The model under review builds one solid part; all positions refer to its coordinate system, in mm. A direction names the side the tool comes from. Coordinates: 2 decimals unless noted, no trailing zeros. Order: outer loops, then holes, each group sorted by start corner. A loop starts at its lowest first (then second) coordinate and runs counter-clockwise, first axis right, second up. Notation, with made-up numbers: (-21, 4.25) -> (12, 4.25) arc R19 ccw to (12, 8.25) -> close; hole circle Ø4 at (7.5, 6.25). An arc over 180 degrees is marked (long way). Use one line per item in the form item = value.
from build123d import *

# Parameters (mm, degrees)
MODEL_W             = 5.5
MODEL_H             = 5.5
BOSS_EXTRUDE1_DEPTH = 6


with BuildPart() as part:
    # Model → Boss-Extrude1 (new body)
    with BuildSketch(Plane.XY):
        with BuildLine():
            Line((3076.532777825, 1463.171342736), (3076.532777825, 1427.171342736))
            Line((3076.532777825, 1427.171342736), (3086.532777825, 1427.171342736))
            Line((3086.532777825, 1427.171342736), (3097.532777825, 1427.171342736))
            Line((3097.532777825, 1427.171342736), (3097.532777825, 1458.171342736))
            Line((3097.532777825, 1458.171342736), (3086.532777825, 1458.171342736))
            Line((3086.532777825, 1458.171342736), (3086.532777825, 1463.171342736))
            ThreePointArc((3086.532777825, 1463.171342736), (3127.532777825, 1504.171342736), (3168.532777825, 1463.171342736))
            Line((3168.532777825, 1463.171342736), (3168.532777825, 1458.171342736))
            Line((3168.532777825, 1458.171342736), (3157.532777825, 1458.171342736))
            Line((3157.532777825, 1458.171342736), (3157.532777825, 1427.171342736))
            Line((3157.532777825, 1427.171342736), (3160.032777825, 1427.171342736))
            Line((3160.032777825, 1427.171342736), (3160.032777825, 1421.171342736))
            Line((3160.032777825, 1421.171342736), (3166.032777825, 1421.171342736))
            Line((3166.032777825, 1421.171342736), (3166.032777825, 1427.171342736))
            Line((3166.032777825, 1427.171342736), (3178.532777825, 1427.171342736))
            Line((3178.532777825, 1427.171342736), (3178.532777825, 1463.171342736))
            ThreePointArc((3178.532777825, 1463.171342736), (3127.532777825, 1514.171342736), (3076.532777825, 1463.171342736))
        make_face()
        with Locations((3163.032777825, 1432.671342736)):
            Rectangle(MODEL_W, MODEL_H, mode=Mode.SUBTRACT)
        with Locations((3163.032777825, 1452.671342736)):
            Rectangle(MODEL_W, MODEL_H, mode=Mode.SUBTRACT)
        with Locations((3092.032777825, 1432.671342736)):
            Rectangle(MODEL_W, MODEL_H, mode=Mode.SUBTRACT)
        with Locations((3092.032777825, 1452.671342736)):
            Rectangle(MODEL_W, MODEL_H, mode=Mode.SUBTRACT)
    extrude(amount=BOSS_EXTRUDE1_DEPTH)


solid = part.part
Item 1: To check wall thickness, follow L1, parallel to X at y = 1445, z = 3.3; L2, parallel to Y at x = 3093, z = 0.8; L3, parallel to X at y = 1471.5, z = 1.35. State the ranges of each line that lie inside material, in increasing order. Write a range as from..to.
Results found:
L1 = 3076.53..3097.53, 3157.53..3178.53
L2 = 1427.17..1429.92, 1435.42..1449.92, 1455.42..1458.17, 1485.27..1500.7
L3 = 3077.22..3087.39, 3167.68..3177.85
Item 2: Tool access review of faces 1 (the face through (3160.283, 1453, 3)), 2 (the face through (3076.533, 1445, 3)), 3 (the face through (3159, 1427.171, 3)): name each direction out of +Z, -Z, +X, -X, +Y, -Y from which nothing blocks a thin tool from reaching the whole face with its end or side.
Results found:
face_1 = +Z, -Z
face_2 = +Z, -Z, -X, +Y, -Y
face_3 = +Z, -Z, -X, -Y
Item 3: Clearance check with flat-ended pins moving along their axes: pin 1 (1.8 mm diameter, centred on x = 3164, z = 2, fed in from +Y); pin 2 (1.5 mm diameter, centred on x = 3123.5, z = 2, fed in from +Y); pin 3 (2 mm diameter, centred on x = 3159, z = 2.5, fed in from -Y). State where each tip first meets the part, or that it passes through.
Results found:
pin_1 = 1499.72
pin_2 = 1514.07
pin_3 = 1427.17
Item 4: We need section B-B (z = 4.7). State how many separate pieces and enclosed holes the cut face has, plus the area to 3 significant figures.
Results found:
separate_pieces = 1
enclosed_holes = 4
area = 2,760 mm²
Item 5: We need section C-C (y = 1443.5). Write out the cut boundary in (x, z).
Results found:
outline = (3076.53, 0) -> (3097.53, 0) -> (3097.53, 6) -> (3076.53, 6) -> close; (3157.53, 0) -> (3178.53, 0) -> (3178.53, 6) -> (3157.53, 6) -> close
Item 6: Draft analysis for pull direction X (two halves, no side actions). For faces 4 (the face through (3092, 1455.421, 3)), 5 (the face through (3097, 1454, 0)), 6 (the face through (3094.783, 1453, 3)), 7 (the face through (3178.533, 1445, 3)), state which applies: released by +X, released by -X, zero draft, split by the parting line, or undercut.
Results found:
face_4 = undercut
face_5 = zero draft
face_6 = undercut
face_7 = released by +X
Item 7: We need section A-A (y = 1460). Write out the cut boundary in (x, z).
Results found:
outline = (3076.53, 0) -> (3086.53, 0) -> (3086.53, 6) -> (3076.53, 6) -> close; (3168.53, 0) -> (3178.53, 0) -> (3178.53, 6) -> (3168.53, 6) -> close
Item 8: We need section D-D (x = 3117). Write out the cut boundary in (y, z), plus the area to 3 significant figures.
Results found:
outline = (1502.8, 0) -> (1513.07, 0) -> (1513.07, 6) -> (1502.8, 6) -> close
area = 61.7 mm²
